```python
from build123d import *
from build123d.topology import SkipClean

# Parameters (mm, degrees)
SKETCH1_R           = 55
SKETCH1_R_2         = 52
BOSS_EXTRUDE1_DEPTH = 25
BOSS_EXTRUDE2_START = -27
BOSS_EXTRUDE2_DEPTH = 29
BOSS_EXTRUDE3_START = 2
SKETCH5_R           = 55
SKETCH5_R_2         = 12
BOSS_EXTRUDE3_DEPTH = 2
SKETCH6_R           = 14
SKETCH6_R_2         = 12.000000000000002
BOSS_EXTRUDE4_DEPTH = 50
SKETCH7_R           = 16
SKETCH7_R_2         = 14.000000000000002
BOSS_EXTRUDE5_DEPTH = 3
BOSS_EXTRUDE6_START = -2
SKETCH8_R           = 55
SKETCH8_R_2         = 52
BOSS_EXTRUDE6_DEPTH = 2
SKETCH9_R           = 11.999999999999996
CUT_EXTRUDE1_DEPTH  = 80.00000000000001
CHAMFER1_SIZE       = 2
BOSS_EXTRUDE8_START = -2
SKETCH11_R          = 56.5
SKETCH11_R_2        = 54.99999999999999
BOSS_EXTRUDE8_DEPTH = 4


with BuildPart() as part:
    # Sketch1 → Boss-Extrude1 (new body)
    with BuildSketch(Plane.XY):
        Circle(SKETCH1_R)
        Circle(SKETCH1_R_2, mode=Mode.SUBTRACT)
    extrude(amount=BOSS_EXTRUDE1_DEPTH)

    # Sketch2 → Boss-Extrude2 (add)
    with BuildSketch(Plane.XY.offset(25).offset(BOSS_EXTRUDE2_START)):
        with BuildLine():
            Line((27, 81.28713256522299), (27, 47.91659420284375))
            ThreePointArc((27, 47.91659420284375), (47.486840282335066, 27.74887385102322), (55, 0))
            Line((55, 0), (55, 81.28713256522299))
            Line((55, 81.28713256522299), (27, 81.28713256522299))
        make_face()
    extrude(amount=BOSS_EXTRUDE2_DEPTH)

    # Sketch5 → Boss-Extrude3 (add)
    with BuildSketch(Plane(origin=(0, 0, 0), x_dir=(-1, 0, 0), z_dir=(0, 0, -1)).offset(BOSS_EXTRUDE3_START)):
        Circle(SKETCH5_R)
        Circle(SKETCH5_R_2, mode=Mode.SUBTRACT)
    extrude(amount=-BOSS_EXTRUDE3_DEPTH)

    # Sketch6 → Boss-Extrude4 (add)
    with BuildSketch(Plane.XY):
        with Locations(Location((0, 0, 0), (0, 0, 180))):
            Circle(SKETCH6_R)
        Circle(SKETCH6_R_2, mode=Mode.SUBTRACT)
    extrude(amount=BOSS_EXTRUDE4_DEPTH)

    # Sketch7 → Boss-Extrude5 (add)
    with BuildSketch(Plane.XY):
        with Locations(Location((0, 0, 0), (0, 0, 180))):
            Circle(SKETCH7_R)
        Circle(SKETCH7_R_2, mode=Mode.SUBTRACT)
    extrude(amount=BOSS_EXTRUDE5_DEPTH)

    # Sketch8 → Boss-Extrude6 (add)
    with BuildSketch(Plane.XY.offset(25).offset(BOSS_EXTRUDE6_START)):
        Circle(SKETCH8_R)
        Circle(SKETCH8_R_2, mode=Mode.SUBTRACT)
    extrude(amount=BOSS_EXTRUDE6_DEPTH)

    # Sketch9 → Cut-Extrude1 (cut)
    with BuildSketch(Plane(origin=(0, 81.28713256522299, 0), x_dir=(1, 0, 0), z_dir=(0, 1, 0))):
        with Locations(Location((41, -12.5, 0), (0, 0, 270))):
            Circle(SKETCH9_R)
    extrude(amount=-CUT_EXTRUDE1_DEPTH, mode=Mode.SUBTRACT)

    # Chamfer1
    chamfer1_edges = [part.edges().sort_by_distance(p)[0] for p in [
        (55, 81.28713256522299, 12.5),
        (27, 81.28713256522299, 12.5),
    ]]
    chamfer(chamfer1_edges, length=CHAMFER1_SIZE)

    # Sketch11 → Boss-Extrude8 (add)
    with SkipClean():  # the faces are left unmerged after this step: merging them gives an invalid solid
        with BuildSketch(Plane.XY.offset(25).offset(BOSS_EXTRUDE8_START)):
            Circle(SKETCH11_R)
            Circle(SKETCH11_R_2, mode=Mode.SUBTRACT)
        extrude(amount=BOSS_EXTRUDE8_DEPTH)


solid = part.part
```
Design review of the part built by this model. Coordinates are the model's own, in mm. A direction names the side the tool comes from. Round coordinates to 2 decimals unless told otherwise and drop trailing zeros. Write each loop counter-clockwise with the first axis right and the second up, starting at its lowest first coordinate (ties: lowest second). Pieces come first, ordered by that corner, then holes.
Item 1: We need section D-D on x = -43. Write out the cut boundary in (y, z).
Item 2: For faces 1 (the flat face through (0.07, 14.15, 3)), 2 (the flat face through (6.3, -10.4, 50)), 3 (the flat face through (13, -1, -2)), 4 (the cylindrical face through (41.625, 35.95, 23.573)), 5 (the flat face through (41, 37, 23)), list the 3-axis set-ups (+Z, -Z, +X, -X, +Y, -Y) from which the entire face can be reached by the end or side of a thin tool; tool diameter is ignored.
Item 3: We need section A-A on x = 0. Write out the cut boundary in (y, z).
Item 4: Clearance check with flat-ended pins moving along their axes: pin 1 Ø23 at (y, z) = (62, 7) entering from -X; pin 2 Ø1.5 at (x, z) = (-39.5, 21) entering from +Y; pin 3 Ø1.5 at (y, z) = (31.5, 26) entering from -X. State where each tip first meets the part, or that it passes through.
Item 5: We need section B-B on z = 6. Write out the cut boundary in (x, y), and give its area (3 significant figures).
Item 6: The part is to be moulded in two halves that separate along Y. For faces 6 (the cylindrical face through (-46.44, -29.47, 10.32)), 7 (the cylindrical face through (-41.265, -31.641, 12.325)), 8 (the flat face through (-37.9, -41.6, 23)), say which applies: +Y half, -Y half, draft (parallel to the pull), parting line (faces both ways), or undercut.
Item 7: For probe 1 along Y at (x, z) = (0, 18.5); probe 2 along X at (y, z) = (0, 26), list the stretches that pass through material, from the lowest coordinate up.
Returned:
1. outline: (-36.65, 23) - (-34.29, 23) - (-34.29, -2) - (34.29, -2) - (34.29, 23) - (36.65, 23) - (36.65, 27) - (34.29, 27) - (34.29, 25) - (29.24, 25) - (29.24, 0) - (-29.24, 0) - (-29.24, 25) - (-34.29, 25) - (-34.29, 27) - (-36.65, 27) - close
2. face 1: +Z
2. face 2: +Z, +X, -X, +Y, -Y
2. face 3: -Z, +X, -X, +Y, -Y
2. face 4: none
2. face 5: +Y
3. outline: (-56.5, 23) - (-55, 23) - (-55, -2) - (-12, -2) - (-12, 50) - (-14, 50) - (-14, 3) - (-16, 3) - (-16, 0) - (-52, 0) - (-52, 25) - (-55, 25) - (-55, 27) - (-56.5, 27) - close; (12, -2) - (55, -2) - (55, 23) - (56.5, 23) - (56.5, 27) - (55, 27) - (55, 25) - (52, 25) - (52, 0) - (16, 0) - (16, 3) - (14, 3) - (14, 50) - (12, 50) - close
4. pin 1: stops at x = -21.79
4. pin 2: stops at y = 39.03
4. pin 3: stops at x = -47.4
5. outline: circle Ø28 at (0, 0); (27, 47.92) arc R55 ccw (long way) to (55, 0) - (55, 79.29) - (53, 81.29) - (51.09, 81.29) - (51.09, 9.7) arc R52 cw (long way) to (30.91, 41.81) - (30.91, 81.29) - (29, 81.29) - (27, 79.29) - close; hole circle Ø24 at (0, 0)
5. area: 1,460 mm2
6. face 6: parting line
6. face 7: undercut
6. face 8: draft
7. probe 1: y = -55 to -52, -14 to -12, 12 to 14, 52 to 55
7. probe 2: x = -56.5 to -55, -14 to -12, 12 to 14, 55 to 56.5
